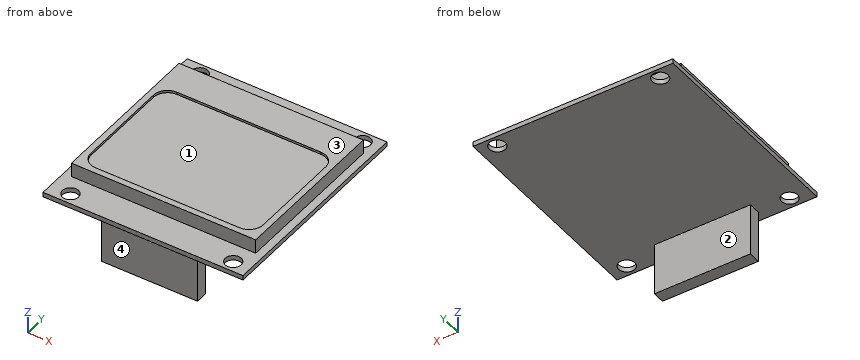
```python
from build123d import *

# Parameters (mm, degrees)
SKETCH_1_W          = 20.32
SKETCH_1_H          = 2.54
EXTRUDE_1_DEPTH     = 11
SKETCH_2_W          = 42.32
SKETCH_2_H          = 45.5
SKETCH_2_R          = 1.7
EXTRUDE_2_DEPTH     = 1
SKETCH_3_W          = 39
SKETCH_3_H          = 34
EXTRUDE_3_DEPTH     = 3
CUT_EXTRUDE_1_DEPTH = 0.5


with BuildPart() as part:
    # 草图1 → 凸台-拉伸1 (new body)
    with BuildSketch(Plane.XY):
        with Locations((34.416985014, 23.365786132)):
            Rectangle(SKETCH_1_W, SKETCH_1_H)
    extrude(amount=EXTRUDE_1_DEPTH)

    # 草图2 → 凸台-拉伸2 (add)
    with BuildSketch(Plane.XY.offset(11)):
        with Locations((34.416985014, 42.762700025)):
            Rectangle(SKETCH_2_W, SKETCH_2_H)
        with Locations((17.486918974, 22.360680721)):
            Circle(SKETCH_2_R, mode=Mode.SUBTRACT)
        with Locations((51.946913894, 22.360680721)):
            Circle(SKETCH_2_R, mode=Mode.SUBTRACT)
        with Locations((17.486918974, 63.235712471)):
            Circle(SKETCH_2_R, mode=Mode.SUBTRACT)
        with Locations((51.946913894, 63.235712471)):
            Circle(SKETCH_2_R, mode=Mode.SUBTRACT)
    extrude(amount=EXTRUDE_2_DEPTH)

    # 草图3 → 凸台-拉伸3 (add)
    with BuildSketch(Plane.XY.offset(12)):
        with Locations((34.416985014, 43.512700025)):
            Rectangle(SKETCH_3_W, SKETCH_3_H)
    extrude(amount=EXTRUDE_3_DEPTH)

    # 草图4 → 切除-拉伸1 (cut)
    with BuildSketch(Plane.XY.offset(15)):
        with BuildLine():
            Line((49.646985014, 27.782700025), (19.186985014, 27.782700025))
            ThreePointArc((19.186985014, 27.782700025), (17.06566467, 28.661379682), (16.186985014, 30.782700025))
            Line((16.186985014, 30.782700025), (16.186985014, 50.512700025))
            ThreePointArc((16.186985014, 50.512700025), (17.06566467, 52.634020369), (19.186985014, 53.512700025))
            Line((19.186985014, 53.512700025), (49.646985014, 53.512700025))
            ThreePointArc((49.646985014, 53.512700025), (51.768305358, 52.634020369), (52.646985014, 50.512700025))
            Line((52.646985014, 50.512700025), (52.646985014, 30.782700025))
            ThreePointArc((52.646985014, 30.782700025), (51.768305358, 28.661379682), (49.646985014, 27.782700025))
        make_face()
    extrude(amount=-CUT_EXTRUDE_1_DEPTH, mode=Mode.SUBTRACT)


solid = part.part
```
Geometry check sheet. Reference: the model listing, model coordinates, mm. Face numbers are marked on the shaded views. A direction names the side the tool comes from. Round coordinates to 2 decimals unless told otherwise and drop trailing zeros. Loops run counter-clockwise (first coordinate to the right, second up) from the corner with the lowest first, then second, coordinate; pieces in that order, holes last. Notation, with made-up numbers: (41.5, -39) - (64.5, -39) arc R16 cw to (64.5, -31) - close; hole circle Ø10 at (24.25, -21.75). An arc over 180 degrees is marked (long way). Write item = value, one per line. Start each with the question number.
1. Mould release check, pull along X, two halves, no side actions. Record for the marked faces 1 and 2: released by +X, released by -X, zero draft, split by the parting line, or undercut.
2. Section check C-C on x = 51.5. Enter the section's corners in (y, z).
3. Thickness scan on line 1 (Y direction, x = 28.5, z = 7.75); line 2 (Z direction, x = 41, y = 34.5); line 3 (X direction, y = 45, z = 13). Record the ranges inside material, lowest first.
4. Section check B-B on y = 62.5. Enter the section's corners in (x, z).
5. Depth check by flat-ended pin: pin 1 (4 mm diameter, centred on y = 47.5, z = 10.5, fed in from -X); pin 2 (21 mm diameter, centred on x = 33, y = 36, fed in from -Z); pin 3 (0.9 mm diameter, centred on x = 40.5, z = 14, fed in from +Y); pin 4 (4.5 mm diameter, centred on x = 17.49, y = 63.24, fed in from +Z). Enter the tip coordinate at first touch or a pass-through.
6. Section check D-D on y = 56.5. Enter the section's corners in (x, z).
7. Section check A-A on x = 37. Enter the section's corners in (y, z), then the cut area to 3 significant figures.
8. Set-up check for the marked faces 3 and 4: record each of +Z, -Z, +X, -X, +Y, -Y from which the full face is reachable in a straight line by a thin tool's end or side.
Working result:
q1.face_1 = undercut
q1.face_2 = zero draft
q2.outline = (20.01, 11) - (20.72, 11) - (20.72, 12) - (20.01, 12) - close; (24, 11) - (61.6, 11) - (61.6, 12) - (60.51, 12) - (60.51, 15) - (52.87, 15) - (52.87, 14.5) - (28.42, 14.5) - (28.42, 15) - (26.51, 15) - (26.51, 12) - (24, 12) - close; (64.88, 11) - (65.51, 11) - (65.51, 12) - (64.88, 12) - close
q3.line_1 = 22.1 to 24.64
q3.line_2 = 11 to 14.5
q3.line_3 = 14.92 to 53.92
q4.outline = (13.26, 11) - (15.95, 11) - (15.95, 12) - (13.26, 12) - close; (19.02, 11) - (50.41, 11) - (50.41, 12) - (19.02, 12) - close; (53.48, 11) - (55.58, 11) - (55.58, 12) - (53.48, 12) - close
q5.pin_1 = 13.26
q5.pin_2 = 11
q5.pin_3 = 60.51
q5.pin_4 = 12
q6.outline = (13.26, 11) - (55.58, 11) - (55.58, 12) - (53.92, 12) - (53.92, 15) - (14.92, 15) - (14.92, 12) - (13.26, 12) - close
q7.outline = (20.01, 11) - (22.1, 11) - (22.1, 0) - (24.64, 0) - (24.64, 11) - (65.51, 11) - (65.51, 12) - (60.51, 12) - (60.51, 15) - (53.51, 15) - (53.51, 14.5) - (27.78, 14.5) - (27.78, 15) - (26.51, 15) - (26.51, 12) - (20.01, 12) - close
q7.area = 163 mm^2
q8.face_3 = +Z, +X, -X, +Y, -Y
q8.face_4 = -Z, +X, -X, -Y
